The drawing under review shows one solid part. Ordinate dimensions are in mm from its lowest x, y, z. A direction names the side the tool comes from. Give positions to 0.01 mm unless a question says otherwise; leave off trailing zeros. Order: outer loops, then holes, each group sorted by start corner. A loop starts at its lowest first (then second) coordinate and runs counter-clockwise, first axis right, second up. Notation, with made-up numbers: (0, 87.5) - (42, 87.5) arc R16 cw to (42, 114.5) - close; hole circle Ø7 at (46, 5). An arc over 180 degrees is marked (long way). Write item = value, one per line. Start each with the question number.
1. We need section B-B, the plane y = 4.5. Give the boundary of the cut face in (x, z).
2. For P1, Ø1, axis at x = 3.5, z = 1, coming from the -Y side, flat-tipped, find the tip position at first contact; note if it passes through.
3. We need section A-A, the plane x = 4. Give the boundary of the cut face in (y, z).
4. Machinability: for the marked faces 1 and 2, which of the approach directions +Z, -Z, +X, -X, +Y, -Y give a long, thin tool a straight path to every point of the face, cutting with its end or side? Answer none if there is none.
5. Wall thickness on probe 1 along Y at (x, z) = (5.25, 5.6); probe 2 along Y at (x, z) = (6.5, 7.5); probe 3 along Z at (x, y) = (1.75, 1.5): over which ranges is each line inside the solid? List them lowest first.
6. We need section D-D, the plane x = 7.25. Give the boundary of the cut face in (y, z).
7. We need section C-C, the plane z = 3.5. Give the boundary of the cut face in (x, y).
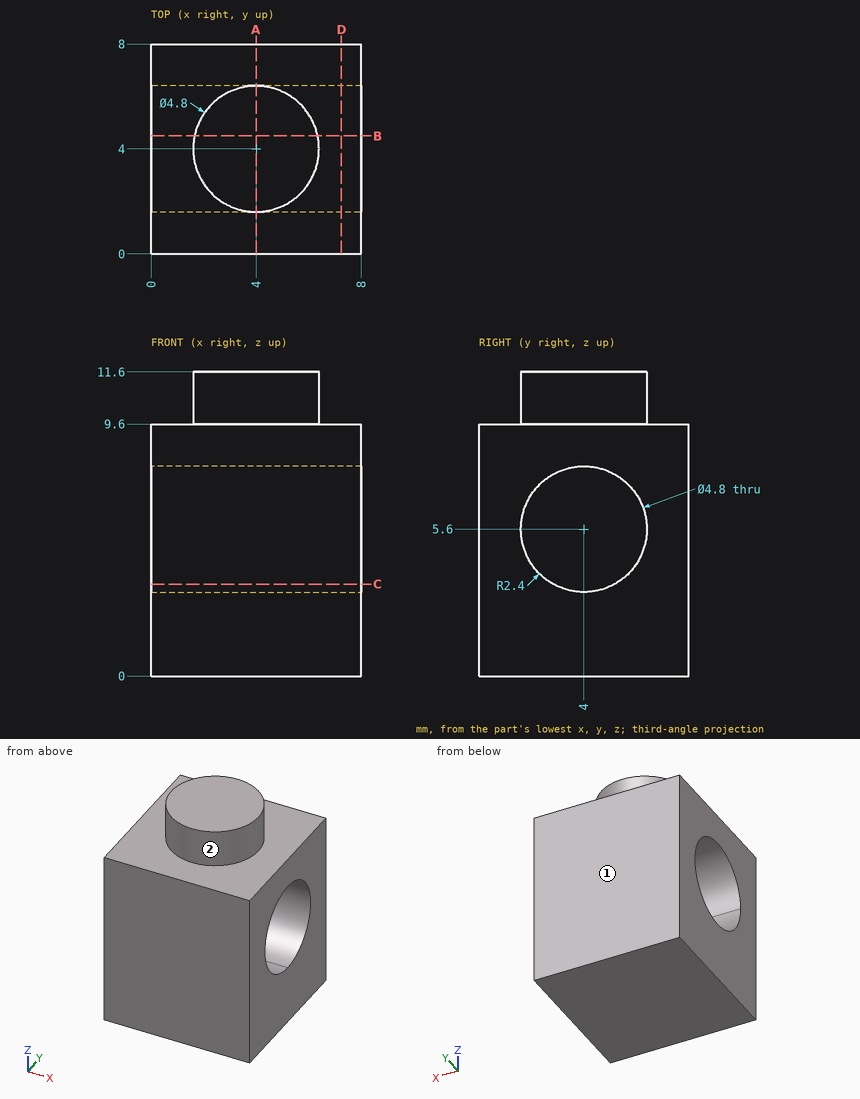
Model answer:
q1.outline = (0, 0) - (8, 0) - (8, 3.25) - (0, 3.25) - close; (0, 7.95) - (8, 7.95) - (8, 9.6) - (6.35, 9.6) - (6.35, 11.6) - (1.65, 11.6) - (1.65, 9.6) - (0, 9.6) - close
q2.P1 = 0
q3.outline = (0, 0) - (8, 0) - (8, 9.6) - (6.4, 9.6) - (6.4, 11.6) - (1.6, 11.6) - (1.6, 9.6) - (0, 9.6) - close; hole (1.6, 5.6) arc R2.4 ccw to (4, 3.2) arc R2.4 ccw (long way) to start
q4.face_1 = +Z, -Z, +X, -X, +Y
q4.face_2 = +Z
q5.probe_1 = 0 to 1.6, 6.4 to 8
q5.probe_2 = 0 to 2.53, 5.47 to 8
q5.probe_3 = 0 to 9.6
q6.outline = (0, 0) - (8, 0) - (8, 9.6) - (0, 9.6) - close; hole (1.6, 5.6) arc R2.4 ccw to (4, 3.2) arc R2.4 ccw (long way) to start
q7.outline = (0, 0) - (8, 0) - (8, 2.84) - (0, 2.84) - close; (0, 5.16) - (8, 5.16) - (8, 8) - (0, 8) - close
